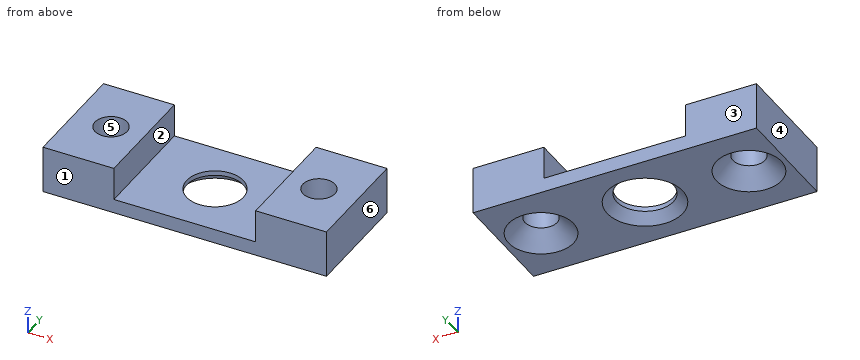
Autodesk Inventor part; units mm, degrees
ref_plane "YZ Plane" through (0, 0, 0) normal (1, 0, 0) x (0, 1, 0)
ref_plane "XZ Plane" through (0, 0, 0) normal (0, 1, 0) x (-1, 0, 0)
ref_plane "XY Plane" through (0, 0, 0) normal (0, 0, 1) x (1, 0, 0)
sketch "Skizze1" plane through (0, 0, 0) normal (0, 0, 1) x (1, 0, 0)
  line L0 (-21, 0) -> (21, 0)
  line L1 (0, -8.4) -> (0, 8.4)
  line L2 (-15, 6) -> (15, 6)
  line L3 (15, 6) -> (15, -6)
  line L4 (15, -6) -> (-15, -6)
  line L5 (-15, -6) -> (-15, 6)
  point P0 (0, 0)
  dimension "d0" = 12
  dimension "d1" = 30
extrude "Extrusion1" add sketch "Skizze1" along normal blind 5
sketch "Skizze2" plane through (0, 0, 5) normal (0, 0, 1) x (1, 0, 0)
  line L0 (15, 6) -> (-15, 6)
  line L1 (-15, -6) -> (15, -6)
  line L2 (-21, 0) -> (21, 0)
  line L3 (0, -8.4) -> (0, 8.4)
  line L4 (-7.5, 6) -> (7.5, 6)
  line L5 (7.5, 6) -> (7.5, -6)
  line L6 (7.5, -6) -> (-7.5, -6)
  line L7 (-7.5, -6) -> (-7.5, 6)
  point P0 (0, 0)
  dimension "d4" = 15
extrude "Extrusion2" cut sketch "Skizze2" against normal blind 3.5
sketch "Skizze3" plane through (0, 0, 0) normal (0, 0, -1) x (-1, 0, 0)
  line L0 (21, 0) -> (-21, 0)
  line L1 (0, -8.4) -> (0, 8.4)
  point P0 (0, 0)
  point P1 (-11, 0)
  point P2 (11, 0)
  dimension "d7" = 22
hole "Bohrung1" at (11, 0, 0) at (-11, 0, 0) direction (0, 0, 1) diameter 3.4 end through all countersink diameter 6.9 countersink angle 90
sketch "Skizze4" plane through (0, 0, 1.5) normal (0, 0, 1) x (1, 0, 0)
  point P0 (0, 0)
  point P1 (0, 0)
hole "Bohrung2" at (0, 0, 1.5) direction (0, 0, -1) diameter 6 end through all
chamfer "Fase1" distance 1 angle 45 1 edges at (0, 3, 0)
properties part number "13_1087_037"
CAD build for the part. Positions are in the model's coordinates, mm. Face numbers are marked on the shaded views. A direction names the side the tool comes from. Give positions to 0.01 mm unless a question says otherwise; leave off trailing zeros. Order: outer loops, then holes, each group sorted by start corner. A loop starts at its lowest first (then second) coordinate and runs counter-clockwise, first axis right, second up. Notation, with made-up numbers: (-26, 38.5) -> (-16, 38.5) arc R18 ccw to (-16, 49.5) -> close; hole circle Ø6 at (-12.75, 17.25). An arc over 180 degrees is marked (long way). Return JSON: item names as keys, results as strings.
Q1. Saw through at B-B (x = -11). Write the cut outline in (y, z).
Working result:
{"outline": "(-6, 0) -> (-3.45, 0) -> (-1.7, 1.75) -> (-1.7, 5) -> (-6, 5) -> close; (1.7, 1.75) -> (3.45, 0) -> (6, 0) -> (6, 5) -> (1.7, 5) -> close"}
Q2. Saw through at C-C (y = 0). Write the cut outline in (x, z).
Working result:
{"outline": "(-15, 0) -> (-14.45, 0) -> (-12.7, 1.75) -> (-12.7, 5) -> (-15, 5) -> close; (-9.3, 1.75) -> (-7.55, 0) -> (-4, 0) -> (-3, 1) -> (-3, 1.5) -> (-7.5, 1.5) -> (-7.5, 5) -> (-9.3, 5) -> close; (3, 1) -> (4, 0) -> (7.55, 0) -> (9.3, 1.75) -> (9.3, 5) -> (7.5, 5) -> (7.5, 1.5) -> (3, 1.5) -> close; (12.7, 1.75) -> (14.45, 0) -> (15, 0) -> (15, 5) -> (12.7, 5) -> close"}
Q3. Which spindle directions (+Z, -Z, +X, -X, +Y, -Y) get a long thin tool onto all of the face, cutting with end or side? Do the marked faces 1 and 2. Say none if no direction does.
Working result:
{"face 1": "+Z, -Z, +X, -X, -Y", "face 2": "+Z, +Y, -Y"}
Q4. Mould opens along X. For the marked faces 3, 4, 5 and 6 say: pulls with the +X half, pulls with the -X half, needs draft (parallel to the pull), parting line crosses it, or undercut.
Working result:
{"face 3": "needs draft", "face 4": "pulls with the -X half", "face 5": "undercut", "face 6": "pulls with the +X half"}
Q5. Drill centre lines: line 1 (X direction, y = 0, z = 4.3); line 2 (Y direction, x = 11, z = 2.9); line 3 (X direction, y = 0.5, z = 0.8). Where is each one in solid material? Low to high.
Working result:
{"line 1": "-15 to -12.7, -9.3 to -7.5, 7.5 to 9.3, 12.7 to 15", "line 2": "-6 to -1.7, 1.7 to 6", "line 3": "-15 to -13.6, -8.4 to -3.16, 3.16 to 8.4, 13.6 to 15"}
Q6. Saw through at A-A (z = 2.8). Write the cut outline in (x, y), then the cut area to 3 significant figures.
Working result:
{"outline": "(-15, -6) -> (-7.5, -6) -> (-7.5, 6) -> (-15, 6) -> close; (7.5, -6) -> (15, -6) -> (15, 6) -> (7.5, 6) -> close; hole circle Ø3.4 at (-11, 0); hole circle Ø3.4 at (11, 0)", "area": "162 mm²"}
Q7. Saw through at D-D (y = -4.5). Write the cut outline in (x, z).
Working result:
{"outline": "(-15, 0) -> (15, 0) -> (15, 5) -> (7.5, 5) -> (7.5, 1.5) -> (-7.5, 1.5) -> (-7.5, 5) -> (-15, 5) -> close"}
Q8. Flat gauge pins, fed straight in: pin 1 (6 mm diameter, centred on x = 3.5, y = -0.5, fed in from +Z); pin 2 (5.5 mm diameter, centred on x = 11, y = 0, fed in from -Z). Where does each tip first touch, or does it go through?
Working result:
{"pin 1": "z = 1.5", "pin 2": "z = 0.7"}
